Here's how the part is built. I have some questions about the finished solid (model axes, mm). A direction names the side the tool comes from. Coordinates: 2 decimals unless noted, no trailing zeros. Loops run counter-clockwise (first coordinate to the right, second up) from the corner with the lowest first, then second, coordinate; pieces in that order, holes last.
from build123d import *

# Parameters (mm, degrees)
SKETCH_R     = 6.5
PAD_DEPTH    = 3
SKETCH001_R  = 3
POCKET_DEPTH = 3
SKETCH002_W  = 9.5
SKETCH002_H  = 19
PAD001_DEPTH = 1.2
SKETCH004_W  = 5
SKETCH004_H  = 3
PAD002_DEPTH = 0.6
CHAMFER_SIZE = 0.59


with BuildPart() as part:
    # Sketch → Pad (new body)
    with BuildSketch(Plane.XY):
        Circle(SKETCH_R)
    extrude(amount=PAD_DEPTH)

    # Sketch001 (on Face3 of Pad) → Pocket (cut)
    with BuildSketch(Plane.XY.offset(3)):
        Circle(SKETCH001_R)
    extrude(amount=-POCKET_DEPTH, mode=Mode.SUBTRACT)

    # Sketch002 → Pad001 (join)
    with BuildSketch(Plane.XY):
        with Locations((0, -13.5)):
            Rectangle(SKETCH002_W, SKETCH002_H)
    extrude(amount=PAD001_DEPTH)

    # Sketch004 (on Face4 of Pad001) → Pad002 (join)
    with BuildSketch(Plane.XY.offset(1.2)):
        with Locations((0, -12.5)):
            Rectangle(SKETCH004_W, SKETCH004_H)
    extrude(amount=PAD002_DEPTH)

    # Chamfer
    chamfer_edges = [part.edges().sort_by_distance(p)[0] for p in [
        (0, -14, 1.8),
        (0, -11, 1.8),
    ]]
    chamfer(chamfer_edges, length=CHAMFER_SIZE)


solid = part.part
Q1. Suppose I cut it at B-B on y = 0. Write out the boundary of the cut face in (x, z), and give its area (3 significant figures).
Q2. Suppose I cut it at C-C on z = 0.75. Write out the boundary of the cut face in (x, y), and give its area (3 significant figures).
Q3. We'd pull the mould along X, two halves only. Please class faces 1 (the cylindrical face through (-3, 0, 2)), 2 (the flat face through (0, -16, 1.2)), 3 (the flat face through (-4.75, -14, 1)): pulls with the +X half, pulls with the -X half, needs draft (parallel to the pull), parting line crosses it, or undercut.
Q4. For faces 4 (the flat face through (0, -12, 1.8)), 5 (the flat face through (4.75, -14, 1)), 6 (the cylindrical face through (-0.846, 6.445, 1.479)), 7 (the flat face through (3, -1, 3)), which set-ups out of +Z, -Z, +X, -X, +Y, -Y let a thin tool reach every point of the face, with its end or its side?
Q5. Please list where these lines run through material, in increasing order: probe 1 along Y at (x, z) = (-1, 1.75); probe 2 along X at (y, z) = (-1, 1.3); probe 3 along Z at (x, y) = (3.5, -18.25).
Q6. Suppose I cut it at D-D on y = -19.25. Write out the boundary of the cut face in (x, z).
Q7. Will these pins go through, and if not, where does the flat tip stop? P1, Ø0.5, axis at y = -12.5, z = 1.5, coming from the +X side; P2, Ø0.5, axis at x = 1, y = -13, coming from the +Z side; P3, Ø5.5, axis at x = 0, y = 0, coming from the -Z side.
Check values:
1. outline: (-6.5, 0) - (-3, 0) - (-3, 3) - (-6.5, 3) - close; (3, 0) - (6.5, 0) - (6.5, 3) - (3, 3) - close
1. area: 21.0 mm2
2. outline: (-4.75, -23) - (4.75, -23) - (4.75, -4.44) arc R6.5 ccw (long way) to (-4.75, -4.44) - close; hole circle Ø6 at (0, 0)
2. area: 267 mm2
3. face 1: undercut
3. face 2: needs draft
3. face 3: pulls with the -X half
4. face 4: +Z, +X, -X, -Y
4. face 5: +Z, -Z, +X, -Y
4. face 6: +Z
4. face 7: +Z, +X, -X, +Y, -Y
5. probe 1: y = -13.46 to -11.54, -6.42 to -2.83, 2.83 to 6.42
5. probe 2: x = -6.42 to -2.83, 2.83 to 6.42
5. probe 3: z = 0 to 1.2
6. outline: (-4.75, 0) - (4.75, 0) - (4.75, 1.2) - (-4.75, 1.2) - close
7. P1: stops at x = 2.5
7. P2: stops at z = 1.8
7. P3: passes through
